The model under review builds one solid part; all positions refer to its coordinate system, in mm. A direction names the side the tool comes from. Coordinates: 2 decimals unless noted, no trailing zeros. Order: outer loops, then holes, each group sorted by start corner. A loop starts at its lowest first (then second) coordinate and runs counter-clockwise, first axis right, second up. Notation, with made-up numbers: M 41.5,-29.75 L 64.5,-29.75 A22 ccw 64.5,-10.75 Z; hole C 74.5,44 d5. An arc over 180 degrees is marked long. Answer in a Markdown table with one row per item.
from build123d import *

# Parameters (mm, degrees)
EXTRUDE_SKETCH_1_R   = 50
EXTRUDE_SKETCH_1_R_2 = 30.35
EXTRUDE_1_DEPTH      = 30
EXTRUDE_START        = 3
EXTRUDE_SKETCH_2_W   = 16
EXTRUDE_SKETCH_2_H   = 20
EXTRUDE_2_DEPTH      = 24


with BuildPart() as part:
    # Extrude sketch 1 → Extrude 1 (new body)
    with BuildSketch(Plane.XY):
        Circle(EXTRUDE_SKETCH_1_R)
        Circle(EXTRUDE_SKETCH_1_R_2, mode=Mode.SUBTRACT)
    extrude(amount=EXTRUDE_1_DEPTH)


with BuildPart() as body_2:
    # Extrude sketch 2 → Extrude 2 (new body)
    with BuildSketch(Plane.XY.offset(EXTRUDE_START)):
        with Locations((54, 0)):
            Rectangle(EXTRUDE_SKETCH_2_W, EXTRUDE_SKETCH_2_H)
    extrude(amount=EXTRUDE_2_DEPTH)

    # Combine (weld / assembly of features): union part
    add(part.part)


solid = body_2.part
(1) Take a section at A-A (y = 0). Write out the cut boundary in (x, z).
Report:
| item | result |
|---|---|
| outline | M -50,0 L -30.35,0 L -30.35,30 L -50,30 Z; M 30.35,0 L 50,0 L 50,3 L 62,3 L 62,27 L 50,27 L 50,30 L 30.35,30 Z |
(2) Take a section at B-B (x = 0). Write out the cut boundary in (y, z).
Report:
| item | result |
|---|---|
| outline | M -50,0 L -30.35,0 L -30.35,30 L -50,30 Z; M 30.35,0 L 50,0 L 50,30 L 30.35,30 Z |
(3) To check wall thickness, follow line 1 (Y direction, x = 0, z = 6.25); line 2 (X direction, y = 0.5, z = 9.25); line 3 (X direction, y = -17.5, z = 21.25). State the ranges of each line that lie inside material, in increasing order. Write a range as [from, to].
Report:
| item | result |
|---|---|
| line 1 | [-50, -30.35], [30.35, 50] |
| line 2 | [-50, -30.35], [30.35, 62] |
| line 3 | [-46.84, -24.8], [24.8, 46.84] |
(4) Take a section at C-C (z = 8.75). Write out the cut boundary in (x, y), then the cut area to 3 significant figures.
Report:
| item | result |
|---|---|
| outline | M 48.99,-10 L 62,-10 L 62,10 L 48.99,10 A50 ccw long Z; hole C 0,0 d60.7 |
| area | 5,210 mm^2 |
(5) Take a section at D-D (y = -15.5). Write out the cut boundary in (x, z), then the cut area to 3 significant figures.
Report:
| item | result |
|---|---|
| outline | M -47.54,0 L -26.09,0 L -26.09,30 L -47.54,30 Z; M 26.09,0 L 47.54,0 L 47.54,30 L 26.09,30 Z |
| area | 1,290 mm^2 |
(6) Insertion check: P1, Ø1, axis at y = -37, z = 25.5, coming from the +X side; P2, Ø8, axis at y = 10, z = 19.5, coming from the -X side; P3, Ø4, axis at x = 52.5, y = -4, coming from the +Z side. Each pin has a flat end and moves straight along its axis. Give the tip position at first contact, or say it passes through.
Report:
| item | result |
|---|---|
| P1 | x = 34.17 |
| P2 | x = -49.64 |
| P3 | z = 27 |
(7) The part is to be moulded in two halves that separate along X. For faces 3 (the cylindrical face through (47.69, 15.02, 14.79)), 4 (the cylindrical face through (28.948, 9.116, 14.79)), 5 (the flat face through (55, -10, 15)), say which applies: +X half, -X half, draft (parallel to the pull), parting line (faces both ways), or undercut.
Report:
| item | result |
|---|---|
| face 3 | parting line |
| face 4 | undercut |
| face 5 | draft |
(8) Machinability: for faces 1 (the flat face through (55, 10, 15)), 2 (the flat face through (22, -22, 30)), which of the approach directions +Z, -Z, +X, -X, +Y, -Y give a long, thin tool a straight path to every point of the face, cutting with its end or side? Answer none if there is none.
Report:
| item | result |
|---|---|
| face 1 | +Z, -Z, +X, +Y |
| face 2 | +Z, +X, -X, +Y, -Y |
